The listing builds one solid part. Answer for the finished solid, in the listing's coordinates (mm). A direction names the side the tool comes from. Give positions to 0.01 mm unless a question says otherwise; leave off trailing zeros. Write each loop counter-clockwise with the first axis right and the second up, starting at its lowest first coordinate (ties: lowest second). Pieces come first, ordered by that corner, then holes. Notation, with made-up numbers: (52.5, 43.25) - (61.5, 43.25) arc R12 cw to (61.5, 52.25) - close; hole circle Ø8 at (76.5, 23). An arc over 180 degrees is marked (long way). One line per item, written item: value. Start each with the question number.
from build123d import *

# Parameters (mm, degrees)
SKETCH1_W                      = 40.1
SKETCH1_H                      = 40.8
BASE_FLANGE1_DEPTH             = 1.5
EDGE_FLANGE2_STRIP_W           = 9.3
EDGE_FLANGE2_STRIP_H           = 1.5
EDGE_FLANGE2_STRIP_CUT_DEPTH   = 40.1
EDGE_FLANGE2_STRIP_2_W         = 9.3
EDGE_FLANGE2_STRIP_2_H         = 1.5
EDGE_FLANGE2_STRIP_CUT_2_DEPTH = 40.1
EDGE_FLANGE2_DEPTH             = 40.1
EDGE_FLANGE2_BEND_DEPTH        = 40.1
SKETCH23_W                     = 3.15
SKETCH23_H                     = 26.7
CUT_EXTRUDE3_DEPTH             = 19
SKETCH24_R                     = 11
CUT_EXTRUDE4_DEPTH             = 55.364349532
SKETCH26_W                     = 10
SKETCH26_H                     = 37.5
CUT_EXTRUDE5_DEPTH             = 39.944222935
SKETCH27_R                     = 1.45
CUT_EXTRUDE6_DEPTH             = 39.944222935
FILLET1_R                      = 3
FILLET2_R                      = 2
F_2_0MM_DOWEL_HOLE1_D          = 2.2
F_2_0MM_DOWEL_HOLE1_DEPTH      = 1.5
F_2_0MM_DOWEL_HOLE2_D          = 2.2
F_2_0MM_DOWEL_HOLE2_DEPTH      = 1.5
CUT_EXTRUDE7_DEPTH             = 40.93122212
FILLET3_R                      = 2


# Sheet-metal steps are written as plain solids
with BuildPart() as part:
    # Sketch1 → Base-Flange1 (new body)
    with BuildSketch(Plane(origin=(0, 0, 0), x_dir=(1, 0, 0), z_dir=(0, 1, 0))):
        Rectangle(SKETCH1_W, SKETCH1_H)
    extrude(amount=-BASE_FLANGE1_DEPTH)

    # Edge-Flange2 strip (across the edge) → Edge-Flange2 strip cut (cut)
    with BuildSketch(Plane(origin=(-20.05, 0, 20.4), x_dir=(0, 0, -1), z_dir=(1, 0, 0))):
        with Locations((-3, -0.75)):
            Rectangle(EDGE_FLANGE2_STRIP_W, EDGE_FLANGE2_STRIP_H)
    extrude(amount=EDGE_FLANGE2_STRIP_CUT_DEPTH, mode=Mode.SUBTRACT)

    # Edge-Flange2 strip 2 (across the edge) → Edge-Flange2 strip cut 2 (cut)
    with BuildSketch(Plane(origin=(20.05, 0, -20.4), x_dir=(0, 0, 1), z_dir=(-1, 0, 0))):
        with Locations((-3, -0.75)):
            Rectangle(EDGE_FLANGE2_STRIP_2_W, EDGE_FLANGE2_STRIP_2_H)
    extrude(amount=EDGE_FLANGE2_STRIP_CUT_2_DEPTH, mode=Mode.SUBTRACT)

    # Edge-Flange2 section (across the edge) → Edge-Flange2 (add)
    with BuildSketch(Plane(origin=(-20.05, 0, 20.4), x_dir=(0, 0, -1), z_dir=(1, 0, 0))):
        with BuildLine():
            Line((-1.5, 1.65), (-1.5, 25.2))
            Line((-1.5, 25.2), (0, 25.2))
            Line((0, 25.2), (0, 1.65))
            ThreePointArc((0, 1.65), (0.483273811, 0.483273811), (1.65, 0))
            Line((1.65, 0), (1.65, -1.5))
            ThreePointArc((1.65, -1.5), (-0.577386361, -0.577386361), (-1.5, 1.65))
        make_face()
    extrude(amount=EDGE_FLANGE2_DEPTH)

    # Edge-Flange2 section 2 (across the edge) → Edge-Flange2 bend (add)
    with BuildSketch(Plane(origin=(20.05, 0, -20.4), x_dir=(0, 0, 1), z_dir=(-1, 0, 0))):
        with BuildLine():
            Line((-1.5, 1.65), (-1.5, 25.2))
            Line((-1.5, 25.2), (0, 25.2))
            Line((0, 25.2), (0, 1.65))
            ThreePointArc((0, 1.65), (0.483273811, 0.483273811), (1.65, 0))
            Line((1.65, 0), (1.65, -1.5))
            ThreePointArc((1.65, -1.5), (-0.577386361, -0.577386361), (-1.5, 1.65))
        make_face()
    extrude(amount=EDGE_FLANGE2_BEND_DEPTH)

    # Sketch23 → Cut-Extrude3 (cut)
    with BuildSketch(Plane(origin=(20.05, 0, 0), x_dir=(0, 0, -1), z_dir=(1, 0, 0))):
        with Locations((-20.325, 11.85)):
            Rectangle(SKETCH23_W, SKETCH23_H)
        with Locations((20.325, 11.85)):
            Rectangle(SKETCH23_W, SKETCH23_H)
    extrude(amount=-CUT_EXTRUDE3_DEPTH, mode=Mode.SUBTRACT)

    # Sketch24 → Cut-Extrude4 (cut, through all)
    with BuildSketch(Plane(origin=(0, 0, -21.9), x_dir=(-1, 0, 0), z_dir=(0, 0, -1))):
        with Locations((-10.25, 14.1)):
            Circle(SKETCH24_R)
    extrude(amount=-CUT_EXTRUDE4_DEPTH, mode=Mode.SUBTRACT)

    # Sketch26 → Cut-Extrude5 (cut, through all)
    with BuildSketch(Plane(origin=(0, 0, 0), x_dir=(1, 0, 0), z_dir=(0, 1, 0))):
        with Locations((15.05, 0)):
            Rectangle(SKETCH26_W, SKETCH26_H)
    extrude(amount=-CUT_EXTRUDE5_DEPTH, mode=Mode.SUBTRACT)

    # Sketch27 → Cut-Extrude6 (cut, through all)
    with BuildSketch(Plane(origin=(0, 0, 0), x_dir=(1, 0, 0), z_dir=(0, 1, 0))):
        with Locations(Location((-16.55, 14.75, 0), (0, 0, 270))):
            Circle(SKETCH27_R)
        with Locations(Location((6.55, 14.75, 0), (0, 0, 270))):
            Circle(SKETCH27_R)
        with Locations(Location((6.55, -14.75, 0), (0, 0, 270))):
            Circle(SKETCH27_R)
        with Locations(Location((-16.55, -14.75, 0), (0, 0, 270))):
            Circle(SKETCH27_R)
    extrude(amount=-CUT_EXTRUDE6_DEPTH, mode=Mode.SUBTRACT)

    # Fillet1
    fillet1_edges = [part.edges().sort_by_distance(p)[0] for p in [
        (10.05, -0.75, 18.75),
        (10.05, -0.75, -18.75),
    ]]
    fillet(fillet1_edges, radius=FILLET1_R)

    # Fillet2
    fillet2_edges = [part.edges().sort_by_distance(p)[0] for p in [
        (1.05, 25.2, -21.15),
        (1.05, 20.129925373, 21.15),
        (1.05, 8.070074627, 21.15),
        (1.05, 20.129925373, -21.15),
        (1.05, 8.070074627, -21.15),
        (-20.05, 25.2, 21.15),
        (-20.05, 25.2, -21.15),
        (1.05, 25.2, 21.15),
    ]]
    fillet(fillet2_edges, radius=FILLET2_R)

    # Ø2.0mm Dowel Hole1
    with Locations(Plane(origin=(0, 0, -21.9), x_dir=(-1, 0, 0), z_dir=(0, 0, -1))):
        with Locations((2.5, 22.7), (17.6, 22.7), (2.5, 7.5), (17.6, 7.5)):
            Hole(F_2_0MM_DOWEL_HOLE1_D / 2, depth=F_2_0MM_DOWEL_HOLE1_DEPTH)

    # Ø2.0mm Dowel Hole2
    with Locations(Plane.XY.offset(21.9)):
        with Locations((-16.95, 15.1), (-9.95, 22.1), (-9.95, 8.1)):
            Hole(F_2_0MM_DOWEL_HOLE2_D / 2, depth=F_2_0MM_DOWEL_HOLE2_DEPTH)

    # Sketch32 → Cut-Extrude7 (cut, through all)
    with BuildSketch(Plane.XZ.offset(1.5)):
        with BuildLine():
            Line((-20.05, 4.5), (-20.05, -4.5))
            Line((-20.05, -4.5), (-15, -4.5))
            ThreePointArc((-15, -4.5), (-14.292893219, -4.207106781), (-14, -3.5))
            Line((-14, -3.5), (-14, 3.5))
            ThreePointArc((-14, 3.5), (-14.292893219, 4.207106781), (-15, 4.5))
            Line((-15, 4.5), (-20.05, 4.5))
        make_face()
    extrude(amount=-CUT_EXTRUDE7_DEPTH, mode=Mode.SUBTRACT)

    # Fillet3
    fillet3_edges = [part.edges().sort_by_distance(p)[0] for p in [
        (-20.05, -0.75, -4.5),
        (-20.05, -0.75, 4.5),
    ]]
    fillet(fillet3_edges, radius=FILLET3_R)


solid = part.part
Item 1: Find section A-A on x = -9.95. Determine the outline of the cut face in (y, z), plus the area to 3 significant figures.
Item 2: Find section C-C on y = 22.1. Determine the outline of the cut face in (x, z).
Item 3: Find section B-B on z = -14.75. Determine the outline of the cut face in (x, y), plus the area to 4 significant figures.
Item 4: For faces 4 (the flat face through (-5, 0, 0)), 5 (the cylindrical face through (-19.48, -0.74, -5.1)), 6 (the cylindrical face through (0.98, 8.02, 21.14)), 7 (the flat face through (1.05, 3, 21)), determine the directions among +Z, -Z, +X, -X, +Y, -Y from which every point of the face is accessible in a straight line to the end or side of a thin tool.
Item 5: Each of these flat-tipped pins is pushed along its axis until it touches: pin 1 Ø1.6 at (y, z) = (1.5, 21) entering from +X; pin 2 Ø4 at (x, z) = (-3, -8.5) entering from +Y; pin 3 Ø1.2 at (x, y) = (-16.5, -0.5) entering from +Z; pin 4 Ø1 at (x, y) = (2, 2) entering from -Z. Where does it stop, or does it pass through?
Item 6: The mould has two halves that part along Z. Classify faces 1 (the flat face through (4, -1, -18.75)), 2 (the flat face through (-17, -1, -4.5)), 3 (the cylindrical face through (-0.75, 14.02, -21.16)): +Z half, -Z half, draft (parallel to the pull), parting line (faces both ways), or undercut.
Item 7: Straight lines are drawn through the part: line 1 along X through (y, z) = (-0.4, -14.75); line 2 along Z through (x, y) = (-7, 22.5); line 3 along Y through (x, z) = (-17.6, -21.6). For each, find the intervals that lie inside material, in ascending order.
Item 8: Find section D-D on x = -2. Determine the outline of the cut face in (y, z), plus the area to 3 significant figures.
Values:
1. outline: (-1.5, -18.75) arc R3.15 ccw to (1.65, -21.9) - (25.2, -21.9) - (25.2, -20.4) - (1.65, -20.4) arc R1.65 cw to (0, -18.75) - (0, 18.75) arc R1.65 cw to (1.65, 20.4) - (7, 20.4) - (7, 21.9) - (1.65, 21.9) arc R3.15 ccw to (-1.5, 18.75) - close; (9.2, 20.4) - (21, 20.4) - (21, 21.9) - (9.2, 21.9) - close; (23.2, 20.4) - (25.2, 20.4) - (25.2, 21.9) - (23.2, 21.9) - close
1. area: 132 mm^2
2. outline: (-20.05, -21.9) - (-18.52, -21.9) - (-18.52, -20.4) - (-20.05, -20.4) - close; (-20.05, 20.4) - (-11.05, 20.4) - (-11.05, 21.9) - (-20.05, 21.9) - close; (-16.68, -21.9) - (-3.42, -21.9) - (-3.42, -20.4) - (-16.68, -20.4) - close; (-8.85, 20.4) - (1.05, 20.4) - (1.05, 21.9) - (-8.85, 21.9) - close; (-1.58, -21.9) - (1.05, -21.9) - (1.05, -20.4) - (-1.58, -20.4) - close
3. outline: (-20.05, -1.5) - (-18, -1.5) - (-18, 0) - (-20.05, 0) - close; (-15.1, -1.5) - (5.1, -1.5) - (5.1, 0) - (-15.1, 0) - close; (8, -1.5) - (10.05, -1.5) - (10.05, 0) - (8, 0) - close
3. area: 36.45 mm^2
4. face 4: +X, -X, +Y
4. face 5: -X, +Y, -Y
4. face 6: +Z, -Z, +X
4. face 7: +Z, +X, +Y, -Y
5. pin 1: x = 1.05
5. pin 2: y = 0
5. pin 3: z = 21.49
5. pin 4: through
6. face 1: -Z half
6. face 2: undercut
6. face 3: draft
7. line 1: -20.05 to -18, -15.1 to 5.1, 8 to 10.05
7. line 2: -21.9 to -20.4, 20.4 to 21.9
7. line 3: 0.31 to 6.4, 8.6 to 21.6, 23.8 to 25.2
8. outline: (-1.5, -18.75) arc R3.15 ccw to (1.65, -21.9) - (6.52, -21.9) - (6.52, -20.4) - (1.65, -20.4) arc R1.65 cw to (0, -18.75) - (0, 18.75) arc R1.65 cw to (1.65, 20.4) - (25.2, 20.4) - (25.2, 21.9) - (1.65, 21.9) arc R3.15 ccw to (-1.5, 18.75) - close; (8.48, -21.9) - (21.72, -21.9) - (21.72, -20.4) - (8.48, -20.4) - close; (23.68, -21.9) - (25.2, -21.9) - (25.2, -20.4) - (23.68, -20.4) - close
8. area: 132 mm^2
